from build123d import *

# Parameters (mm, degrees)
SKETCH1_R           = 1.4224
BOSS_EXTRUDE1_DEPTH = 4
SKETCH3_R           = 3.5
SKETCH3_R_2         = 1.4224
BOSS_EXTRUDE2_DEPTH = 20


with BuildPart() as part:
    # Sketch1 → Boss-Extrude1 (new body)
    with BuildSketch(Plane.XY.offset(206.266714263)):
        with BuildLine():
            Line((164.026557277, 113.230165261), (164.026557277, 189.230165261))
            ThreePointArc((164.026557277, 189.230165261), (163.001431011, 191.705038995), (160.526557277, 192.730165261))
            Line((160.526557277, 192.730165261), (108.526557277, 192.730165261))
            ThreePointArc((108.526557277, 192.730165261), (106.051683543, 191.705038995), (105.026557277, 189.230165261))
            Line((105.026557277, 189.230165261), (105.026557277, 113.230165261))
            ThreePointArc((105.026557277, 113.230165261), (106.051683543, 110.755291526), (108.526557277, 109.730165261))
            Line((108.526557277, 109.730165261), (160.526557277, 109.730165261))
            ThreePointArc((160.526557277, 109.730165261), (163.001431011, 110.755291526), (164.026557277, 113.230165261))
        make_face()
        with Locations((160.526557277, 113.230165261)):
            Circle(SKETCH1_R, mode=Mode.SUBTRACT)
        with Locations((108.526557277, 113.230165261)):
            Circle(SKETCH1_R, mode=Mode.SUBTRACT)
        with Locations((160.526557277, 189.230165261)):
            Circle(SKETCH1_R, mode=Mode.SUBTRACT)
        with Locations((108.526557277, 189.230165261)):
            Circle(SKETCH1_R, mode=Mode.SUBTRACT)
    extrude(amount=BOSS_EXTRUDE1_DEPTH)

    # Sketch3 → Boss-Extrude2 (add)
    with BuildSketch(Plane(origin=(0, 0, 206.266714263), x_dir=(-1, 0, 0), z_dir=(0, 0, -1))):
        with Locations((-108.526557277, 189.230165261)):
            Circle(SKETCH3_R)
        with Locations((-108.526557277, 189.230165261)):
            Circle(SKETCH3_R_2, mode=Mode.SUBTRACT)
        with Locations((-160.526557277, 189.230165261)):
            Circle(SKETCH3_R)
        with Locations((-160.526557277, 189.230165261)):
            Circle(SKETCH3_R_2, mode=Mode.SUBTRACT)
        with Locations((-160.526557277, 113.230165261)):
            Circle(SKETCH3_R)
        with Locations((-160.526557277, 113.230165261)):
            Circle(SKETCH3_R_2, mode=Mode.SUBTRACT)
        with Locations((-108.526557277, 113.230165261)):
            Circle(SKETCH3_R)
        with Locations((-108.526557277, 113.230165261)):
            Circle(SKETCH3_R_2, mode=Mode.SUBTRACT)
    extrude(amount=BOSS_EXTRUDE2_DEPTH)


solid = part.part
CAD build for the part. Positions are in the model's coordinates, mm. Coordinates: 2 decimals unless noted, no trailing zeros. Order: outer loops, then holes, each group sorted by start corner. A loop starts at its lowest first (then second) coordinate and runs counter-clockwise, first axis right, second up.
Item 1: Band-saw the part on C-C on y = 133.5. List the corners of the cut face in (x, z), plus the area to 3 significant figures.
Check sheet entries:
outline: (105.03, 206.27) - (164.03, 206.27) - (164.03, 210.27) - (105.03, 210.27) - close
area: 236 mm2
Item 2: Band-saw the part on D-D on x = 158. List the corners of the cut face in (y, z).
Check sheet entries:
outline: (109.73, 206.27) - (110.81, 206.27) - (110.81, 186.27) - (115.65, 186.27) - (115.65, 206.27) - (186.81, 206.27) - (186.81, 186.27) - (191.65, 186.27) - (191.65, 206.27) - (192.73, 206.27) - (192.73, 210.27) - (109.73, 210.27) - close
Item 3: Band-saw the part on B-B on x = 138.5. List the corners of the cut face in (y, z).
Check sheet entries:
outline: (109.73, 206.27) - (192.73, 206.27) - (192.73, 210.27) - (109.73, 210.27) - close
Item 4: Drill centre lines: L1, parallel to X at y = 114.5, z = 195.5; L2, parallel to Y at x = 109, z = 190; L3, parallel to Z at x = 151.5, y = 165. Where is each one in solid material? Low to high.
Check sheet entries:
L1: x = 105.27 to 107.89, 109.17 to 111.79, 157.27 to 159.89, 161.17 to 163.79
L2: y = 109.76 to 111.89, 114.57 to 116.7, 185.76 to 187.89, 190.57 to 192.7
L3: z = 206.27 to 210.27
Item 5: Pin check, flat tips, straight feed: pin 1 Ø3.5 at (x, y) = (108.53, 189.23) entering from +Z; pin 2 Ø2 at (x, y) = (116.5, 172.5) entering from -Z. Stop position of each tip, or through.
Check sheet entries:
pin 1: stops at z = 210.27
pin 2: stops at z = 206.27
Item 6: Two-plate mould, pull along X, no slides. Class faces 1 (the face through (164.027, 151, 208)), 2 (the face through (107, 112.5, 186.267)), 3 (the face through (134, 152, 206.267)): +X half, -X half, draft (parallel to the pull), parting line (faces both ways), or undercut.
Check sheet entries:
face 1: +X half
face 2: draft
face 3: undercut
Item 7: Band-saw the part on A-A on z = 202. List the corners of the cut face in (x, y), plus the area to 3 significant figures.
Check sheet entries:
outline: circle Ø7 at (108.53, 113.23); circle Ø7 at (108.53, 189.23); circle Ø7 at (160.53, 113.23); circle Ø7 at (160.53, 189.23); hole circle Ø2.84 at (108.53, 113.23); hole circle Ø2.84 at (108.53, 189.23); hole circle Ø2.84 at (160.53, 113.23); hole circle Ø2.84 at (160.53, 189.23)
area: 129 mm2
